```python
from build123d import *

# Parameters (mm, degrees)
SKETCH1_R                = 2.5
FORMABASE_DEPTH          = 2.1
FILLET1_R                = 0.5
BOSS_EXTRUDE2_DEPTH      = 2.9
BOSS_EXTRUDE2_DEPTH_BACK = 2.9
BOSS_EXTRUDE2_START      = -5.5
SKETCH3_W                = 1.7
SKETCH3_H                = 2.2
CUT_EXTRUDE1_DEPTH       = 11.094552987
SKETCH4_R                = 2.5
SKETCH4_R_2              = 2.25
SKETCH4_R_3              = 0.5
BOSS_EXTRUDE3_DEPTH      = 0.6
SKETCH5_R                = 0.5
BOSS_EXTRUDE4_DEPTH      = 0.4
SKETCH6_R                = 2.25
CUT_EXTRUDE2_DEPTH       = 0.01


with BuildPart() as part:
    # Sketch1 → FormaBase (new body)
    # profile 1 of 2: a face of its own
    with BuildSketch(Plane(origin=(0, 0, 0), x_dir=(1, 0, 0), z_dir=(0, 1, 0))):
        Polygon((-5, -6), (5, -6), (5.5, -5.5), (5.5, 2), (2.5, 6), (-2.5, 6), (-5.5, 2), (-5.5, -5.5), align=None)
        Circle(SKETCH1_R, mode=Mode.SUBTRACT)
    # profile 2 of 2: a face of its own
    with BuildSketch(Plane(origin=(0, 0, 0), x_dir=(1, 0, 0), z_dir=(0, 1, 0))):
        Circle(SKETCH1_R)
        with BuildLine():
            ThreePointArc((-1.732050808, 1), (0, -2), (1.732050808, 1))
            Line((1.732050808, 1), (-1.732050808, 1))
        make_face(mode=Mode.SUBTRACT)
    extrude(amount=FORMABASE_DEPTH)

    # Fillet1
    fillet1_edges = [part.edges().sort_by_distance(p)[0] for p in [
        (-5.5, 1.05, -2),
        (-2.5, 1.05, -6),
        (2.5, 1.05, -6),
        (5.5, 1.05, -2),
    ]]
    fillet(fillet1_edges, radius=FILLET1_R)

    # Sketch2 → Boss-Extrude2 (add, two sides: drawn at the far end of the back side and taken through both)
    with BuildSketch(Plane(origin=(5.5, 0, 0), x_dir=(0, 0, -1), z_dir=(1, 0, 0)).offset(BOSS_EXTRUDE2_START - BOSS_EXTRUDE2_DEPTH_BACK)):
        with BuildLine():
            Line((-8.2, 0), (-7.05, 0))
            ThreePointArc((-7.05, 0), (-6.979289322, 0.029289322), (-6.95, 0.1))
            Line((-6.95, 0.1), (-6.95, 0.5))
            ThreePointArc((-6.95, 0.5), (-6.920710678, 0.570710678), (-6.85, 0.6))
            Line((-6.85, 0.6), (-6, 0.6))
            Line((-6, 0.6), (-6, 0.8))
            Line((-6, 0.8), (-7.05, 0.8))
            ThreePointArc((-7.05, 0.8), (-7.120710678, 0.770710678), (-7.15, 0.7))
            Line((-7.15, 0.7), (-7.15, 0.2))
            Line((-7.15, 0.2), (-8.2, 0.2))
            Line((-8.2, 0.2), (-8.2, 0))
        make_face()
        Polygon((6, 0.8), (6, 0), (6.7, 0), (6.7, 0.2), (6.1, 0.2), (6.1, 0.8), align=None)
    extrude(amount=BOSS_EXTRUDE2_DEPTH + BOSS_EXTRUDE2_DEPTH_BACK)

    # Sketch3 → Cut-Extrude1 (cut, through all)
    with BuildSketch(Plane(origin=(0, 2.1, 0), x_dir=(1, 0, 0), z_dir=(0, 1, 0))):
        with Locations((-1.25, -7.1)):
            Rectangle(SKETCH3_W, SKETCH3_H)
        with Locations((1.25, -7.1)):
            Rectangle(SKETCH3_W, SKETCH3_H)
        Polygon((-2.1, 6), (-0.4, 6), (-0.4, 6.7), (-2.9, 6.7), (-2.9, 6), (-2.25, 6), align=None)
        Polygon((0.4, 6.7), (0.4, 6), (2.1, 6), (2.25, 6), (2.9, 6), (2.9, 6.7), align=None)
    extrude(amount=-CUT_EXTRUDE1_DEPTH, mode=Mode.SUBTRACT)

    # Sketch4 → Boss-Extrude3 (add)
    # profile 1 of 3: a face of its own
    with BuildSketch(Plane.XZ):
        with Locations(Location((0, 0, 0), (0, 0, 90))):
            Circle(SKETCH4_R)
        with Locations(Location((0, 0, 0), (0, 0, 270))):
            Circle(SKETCH4_R_2, mode=Mode.SUBTRACT)
    # profile 2 of 3: a face of its own
    with BuildSketch(Plane.XZ):
        with Locations(Location((4.25, 5.5, 0), (0, 0, 90))):
            Circle(SKETCH4_R_3)
    # profile 3 of 3: a face of its own
    with BuildSketch(Plane.XZ):
        with Locations(Location((-4.25, 5.5, 0), (0, 0, 90))):
            Circle(SKETCH4_R_3)
    extrude(amount=BOSS_EXTRUDE3_DEPTH)

    # Sketch5 → Boss-Extrude4 (add)
    with BuildSketch(Plane.XZ.offset(0.6)):
        with Locations(Location((-4.25, 5.5, 0), (0, 0, 90))):
            Circle(SKETCH5_R)
        with Locations(Location((4.25, 5.5, 0), (0, 0, 90))):
            Circle(SKETCH5_R)
    extrude(amount=BOSS_EXTRUDE4_DEPTH)

    # Sketch6 → Cut-Extrude2 (cut)
    with BuildSketch(Plane(origin=(0, 2.1, 0), x_dir=(1, 0, 0), z_dir=(0, 1, 0))):
        with Locations(Location((0, 0, 0), (0, 0, 90))):
            Circle(SKETCH6_R)
    extrude(amount=-CUT_EXTRUDE2_DEPTH, mode=Mode.SUBTRACT)


solid = part.part
```
The listing builds one solid part. Answer for the finished solid, in the listing's coordinates (mm). A direction names the side the tool comes from. Round coordinates to 2 decimals unless told otherwise and drop trailing zeros. Loops run counter-clockwise (first coordinate to the right, second up) from the corner with the lowest first, then second, coordinate; pieces in that order, holes last. Notation, with made-up numbers: (-11.75, 87.5) - (7.25, 87.5) arc R14 cw to (7.25, 94.5) - close; hole circle Ø1 at (68.5, -13). An arc over 180 degrees is marked (long way). Use one line per item in the form item = value. Start each with the question number.
1. For a pull along X with two mould halves and no side action, classify faces 5 (the face through (-4.3, -1, 5.5)), 6 (the face through (0.676, -0.296, -2.146)), 7 (the face through (5.5, 1, 2)) as pulls with the +X half, pulls with the -X half, needs draft (parallel to the pull), parting line crosses it, or undercut.
2. A tool of negligible diameter and unlimited length cuts with its end or side. For faces 1 (the face through (-4.746, -0.493, 5.435)), 2 (the face through (4.2, -1, 5.5)), 3 (the face through (0, 1, -1)), 4 (the face through (-2.5, 0.6, 6.4)), from which of +Z, -Z, +X, -X, +Y, -Y can it reach the whole face along a straight path? Write none if from no direction.
3. Given pin 1 Ø0.8 at (y, z) = (0, -6) entering from +X; pin 2 Ø0.6 at (y, z) = (0.5, 7) entering from +X; pin 3 Ø5 at (x, z) = (0, 0) entering from -Y; pin 4 Ø6 at (x, z) = (0, 0) entering from +Y, each flat-ended and moving along its own axis, determine where each tip first touches the part or whether it passes through.
4. The part is cut by section A-A on y = 1.75. Determine the outline of the cut face in (x, z).
5. The part is cut by section D-D on z = 4.75. Determine the outline of the cut face in (x, y), then the cut area to 3 significant figures.
6. Consider line 1 (X direction, y = 0.75, z = 0); line 2 (X direction, y = -0.35, z = 0); line 3 (Z direction, x = 0, y = 1.4). Determine where each line is inside the solid, lowest interval first. Write a range as [from, to].
7. The part is cut by section C-C on y = -0.2. Determine the outline of the cut face in (x, z).
Geometry check:
q1.face_5 = needs draft
q1.face_6 = undercut
q1.face_7 = pulls with the +X half
q2.face_1 = -Y
q2.face_2 = +Z, -Z, +X, -X, -Y
q2.face_3 = +Y, -Y
q2.face_4 = +X, -X, -Y
q3.pin_1 = 2.8
q3.pin_2 = 2.9
q3.pin_3 = -0.6
q3.pin_4 = 2.1
q4.outline = (-5.5, -1.83) arc R0.5 ccw to (-5.4, -2.13) - (-2.65, -5.8) arc R0.5 ccw to (-2.25, -6) - (2.25, -6) arc R0.5 ccw to (2.65, -5.8) - (5.4, -2.13) arc R0.5 ccw to (5.5, -1.83) - (5.5, 5.5) - (5, 6) - (-5, 6) - (-5.5, 5.5) - close; hole (-1.73, -1) - (1.73, -1) arc R2 ccw (long way) to start
q5.outline = (-5.5, 0) - (5.5, 0) - (5.5, 2.1) - (-5.5, 2.1) - close
q5.area = 23.1 mm^2
q6.line_1 = [-5.5, -2], [2, 5.5]
q6.line_2 = [-2.5, -2.25], [2.25, 2.5]
q6.line_3 = [-6, -1], [2, 6]
q7.outline = circle Ø1 at (-4.25, 5.5); circle Ø5 at (0, 0); circle Ø1 at (4.25, 5.5); hole circle Ø4.5 at (0, 0)
